Geometry: final body of the model. Coordinates: model frame, mm. Face numbers are marked on the shaded views. A direction names the side the tool comes from. Give positions to 0.01 mm unless a question says otherwise; leave off trailing zeros. Order: outer loops, then holes, each group sorted by start corner. A loop starts at its lowest first (then second) coordinate and runs counter-clockwise, first axis right, second up. Notation, with made-up numbers: (52, 19.5) -> (64, 19.5) arc R23 ccw to (64, 41.5) -> close; hole circle Ø2 at (56, 39). An arc over 180 degrees is marked (long way). Answer in a Markdown table with one row per item. Add a question column.
Q1. Contact query for flat-ended pins moving along their axis: P1, Ø4, axis at x = 9, y = 13, coming from the -Z side; P2, Ø4, axis at x = 5, z = -7, coming from the +Y side. Output: stop coordinate, or through.
Q2. Cut plane C-C on z = -6. Return the cut outline in (x, y).
Q3. Cut plane D-D on y = 13.75. Return the cut outline in (x, z), and give its area (3 significant figures).
Q4. Cut plane B-B on y = 2.75. Return the cut outline in (x, z).
Q5. Line query: line 1 along X through (y, z) = (1.8, -7); line 2 along Z through (x, y) = (5, 1.6); line 3 along Y through (x, z) = (9.25, -5). Output: solid intervals per line, ascending. Write a range as from..to.
Q6. Pull-direction query (Z, two-part tool) for the marked faces 1, 2 and 3; classes: +Z half, -Z half, draft (parallel to the pull), parting line (faces both ways), or undercut.
Q7. Cut plane A-A on x = 5. Return the cut outline in (y, z).
Q8. Set-up query: the marked faces 4 and 5. Return all of +Z, -Z, +X, -X, +Y, -Y with unobstructed straight access to the full face (end or side cutting, diameter ignored); none if empty.
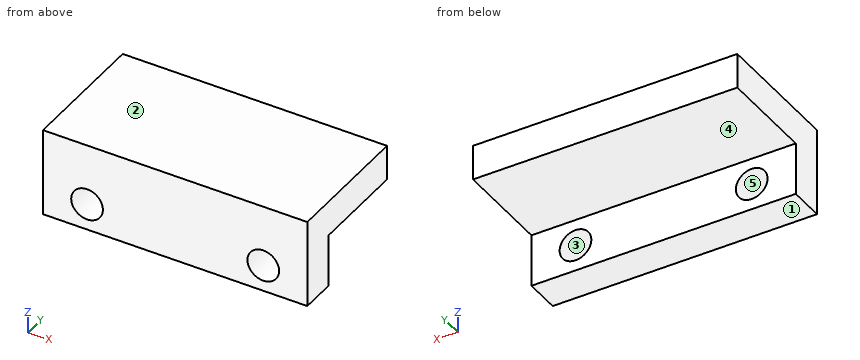
from build123d import *

# Parameters (mm, degrees)
BOSS_EXTRUDE1_DEPTH  = 30
M3_CLEARANCE_HOLE1_D = 3.6


with BuildPart() as part:
    # Sketch1 → Boss-Extrude1 (new body)
    with BuildSketch(Plane(origin=(0, 0, 0), x_dir=(0, 0, -1), z_dir=(1, 0, 0))):
        Polygon((0, 15), (0, 0), (10, 0), (10, 4), (4, 4), (4, 15), align=None)
    extrude(amount=BOSS_EXTRUDE1_DEPTH)

    # M3 Clearance Hole1 (through all)
    with Locations(Plane(origin=(0, 4, 0), x_dir=(1, 0, 0), z_dir=(0, 1, 0))):
        with Locations((5, 7), (25, 7)):
            Hole(M3_CLEARANCE_HOLE1_D / 2)


solid = part.part
Completed:
| question | item | result |
|---|---|---|
| 1 | P1 | stops at z = -4 |
| 1 | P2 | stops at y = 4 |
| 2 | outline | (0, 0) -> (3.5, 0) -> (3.5, 4) -> (0, 4) -> close; (6.5, 0) -> (23.5, 0) -> (23.5, 4) -> (6.5, 4) -> close; (26.5, 0) -> (30, 0) -> (30, 4) -> (26.5, 4) -> close |
| 3 | outline | (0, -4) -> (30, -4) -> (30, 0) -> (0, 0) -> close |
| 3 | area | 120 mm² |
| 4 | outline | (0, -10) -> (30, -10) -> (30, 0) -> (0, 0) -> close; hole circle Ø3.6 at (5, -7); hole circle Ø3.6 at (25, -7) |
| 5 | line 1 | x = 0..3.2, 6.8..23.2, 26.8..30 |
| 5 | line 2 | z = -10..-8.8, -5.2..0 |
| 5 | line 3 | y = 0..4 |
| 6 | face 1 | -Z half |
| 6 | face 2 | +Z half |
| 6 | face 3 | undercut |
| 7 | outline | (0, -10) -> (4, -10) -> (4, -8.8) -> (0, -8.8) -> close; (0, -5.2) -> (4, -5.2) -> (4, -4) -> (15, -4) -> (15, 0) -> (0, 0) -> close |
| 8 | face 4 | -Z, +X, -X, +Y |
| 8 | face 5 | +Y, -Y |
